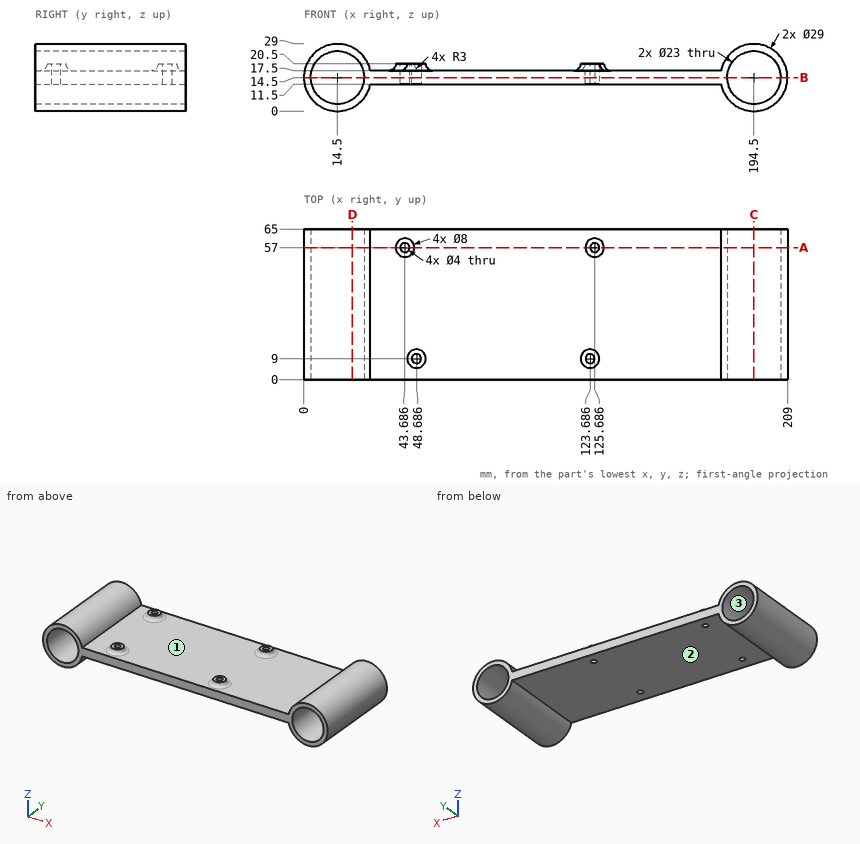
Answer from the drawing. Dimensions are ordinates in mm from the lowest x, y and z of the part. Give positions to 0.01 mm unless a question says otherwise; leave off trailing zeros. Loops run counter-clockwise (first coordinate to the right, second up) from the corner with the lowest first, then second, coordinate; pieces in that order, holes last.
Item 1: The mould has two halves that part along Z. Classify the marked faces 1, 2 and 3: released by +Z, released by -Z, zero draft, split by the parting line, or undercut.
Item 2: The part is cut by section B-B (z = 14.5). Write down the section's boundary in (x, y), and give its area (3 significant figures).
Item 3: The part is cut by section C-C (x = 194.5). Write down the section's boundary in (y, z).
Item 4: Find the intervals of material crossed by line 1 along X through (y, z) = (46.5, 14.5); line 2 along X through (y, z) = (61, 8); line 3 along X through (y, z) = (57, 7.5) (1 decimal), in increasing order.
Item 5: The part is cut by section A-A (y = 57). Give the number of separate pieces and of enclosed holes in the cut face, and give its area (3 significant figures).
Item 6: Each of these flat-tipped pins is pushed along its axis until it touches: pin 1 Ø6.5 at (x, y) = (43.69, 57) entering from -Z; pin 2 Ø2 at (y, z) = (52.5, 9) entering from +X; pin 3 Ø6.5 at (x, y) = (127, 55.5) entering from +Z. Where does it stop, or does it pass through?
Item 7: The part is cut by section D-D (x = 21). Write down the section's boundary in (y, z).
Taken from the geometry:
1. face 1: released by +Z
1. face 2: released by -Z
1. face 3: undercut
2. outline: (0, 0) - (3, 0) - (3, 65) - (0, 65) - close; (26, 0) - (183, 0) - (183, 65) - (26, 65) - close; (206, 0) - (209, 0) - (209, 65) - (206, 65) - close; hole circle Ø4 at (43.69, 57); hole circle Ø4 at (48.69, 9); hole circle Ø4 at (123.69, 9); hole circle Ø4 at (125.69, 57)
2. area: 10,500 mm2
3. outline: (0, 0) - (65, 0) - (65, 3) - (0, 3) - close; (0, 26) - (65, 26) - (65, 29) - (0, 29) - close
4. line 1: x = 0 to 3, 26 to 183, 206 to 209
4. line 2: x = 1.54 to 5.01, 23.99 to 27.46, 181.54 to 185.01, 203.99 to 207.46
4. line 3: x = 1.8 to 5.4, 23.6 to 27.2, 181.8 to 185.4, 203.6 to 207.2
5. separate pieces: 3
5. enclosed holes: 2
5. area: 1,380 mm2
6. pin 1: stops at z = 11.5
6. pin 2: stops at x = 208.28
6. pin 3: stops at z = 20.5
7. outline: (0, 1.54) - (65, 1.54) - (65, 5.01) - (0, 5.01) - close; (0, 23.99) - (65, 23.99) - (65, 27.46) - (0, 27.46) - close
